Can you work these out from the model? Positions are in its coordinate system, mm. Give positions to 0.01 mm unless a question says otherwise; leave off trailing zeros. Order: outer loops, then holes, each group sorted by start corner. A loop starts at its lowest first (then second) coordinate and runs counter-clockwise, first axis right, second up. Notation, with made-up numbers: (-1, 68.5) - (38, 68.5) arc R18 ccw to (38, 99.5) - close; hole circle Ø7 at (76.5, 36.5). An arc over 180 degrees is marked (long way). Return JSON: item names as keys, results as strings.
```python
from build123d import *

# Parameters (mm, degrees)
F0_W     = 300
F0_H     = 400
F1_DEPTH = 19
F3_DEPTH = 19


with BuildPart() as f1:
    # F0 (on Front) → F1 (new body)
    with BuildSketch(Plane.XZ):
        with Locations((-34.205507, 1.972216)):
            Rectangle(F0_W, F0_H)
    extrude(amount=F1_DEPTH)

    # F2 (on face) → F3 (cut)
    with BuildSketch(Plane(origin=(0, 0, 0), x_dir=(-1, 0, 0), z_dir=(0, 1, 0))):
        Polygon((-105.294493, 191.972216), (-105.294493, -176.027784), (-75.294493, -176.027784), (-75.294493, 161.972216), (-63.794493, 161.972216), (-63.794493, -176.027784), (7.705507, -176.027784), (7.705507, 161.972216), (19.205507, 161.972216), (19.205507, -176.027784), (90.705507, -176.027784), (90.705507, 161.972216), (102.205507, 161.972216), (102.205507, -176.027784), (173.705507, -176.027784), (173.705507, 191.972216), (143.705507, 191.972216), (143.705507, -146.027784), (132.205507, -146.027784), (132.205507, 191.972216), (60.705507, 191.972216), (60.705507, -146.027784), (49.205507, -146.027784), (49.205507, 191.972216), (-22.294493, 191.972216), (-22.294493, -146.027784), (-33.794493, -146.027784), (-33.794493, 191.972216), align=None)
    extrude(amount=-F3_DEPTH, mode=Mode.SUBTRACT)


solid = f1.part
```
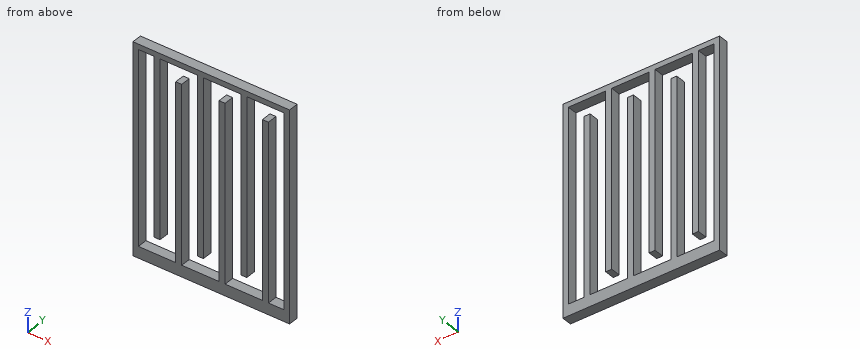
1. Suppose I cut it at A-A (z = 138.5). State how many separate pieces and enclosed holes the cut face has, plus the area to 3 significant figures.
Checks:
{"separate pieces": "8", "enclosed holes": "0", "area": "1,710 mm^2"}
2. If I drill on L1, parallel to Z at x = -119.5, y = -0.75; L2, parallel to Z at x = -52.5, y = -3, over which ranges is the centre line in solid material (lowest first)? Write a range as [from, to].
Checks:
{"L1": "[-198.03, -176.03], [191.97, 201.97]", "L2": "[-198.03, -176.03], [-146.03, 201.97]"}
3. Suppose I cut it at C-C (x = 46). List the corners of the cut face in (y, z) for me, plus the area to 3 significant figures.
Checks:
{"outline": "(-19, -198.03) - (0, -198.03) - (0, -176.03) - (-19, -176.03) - close; (-19, 191.97) - (0, 191.97) - (0, 201.97) - (-19, 201.97) - close", "area": "608 mm^2"}
